Can you work these out from the model? Positions are in its coordinate system, mm. A direction names the side the tool comes from. Give positions to 0.01 mm unless a question says otherwise; leave off trailing zeros. Write each loop counter-clockwise with the first axis right and the second up, starting at its lowest first coordinate (ties: lowest second). Pieces come first, ordered by that corner, then holes.
```python
from build123d import *

# Parameters (mm, degrees)
SKETCH1_W               = 240
SKETCH1_H               = 20
BOSS_EXTRUDE1_DEPTH     = 30
SKETCH2_R               = 5.025
CUT_EXTRUDE1_DEPTH      = 20
SKETCH3_R               = 2.05
CUT_EXTRUDE2_DEPTH      = 30
SKETCH4_W               = 15
SKETCH4_H               = 30
CUT_EXTRUDE3_DEPTH      = 10
CUT_EXTRUDE4_DEPTH      = 2.5
CUT_EXTRUDE5_DEPTH      = 32.5
FILLET1_R               = 10
FILLET2_R               = 10
CHAMFER1_SIZE           = 1
CHAMFER2_SIZE           = 1
SKETCH7_R               = 1.6
CUT_EXTRUDE6_DEPTH      = 32.5
CUT_EXTRUDE7_DEPTH      = 10
SKETCH9_R               = 3
CUT_EXTRUDE8_DEPTH      = 3
FILLET3_R               = 1
CUT_EXTRUDE9_DEPTH      = 3
CUT_EXTRUDE9_DEPTH_BACK = 3
SKETCH10_R              = 3.65
SKETCH11_R              = 1.5
CUT_EXTRUDE10_DEPTH     = 13
SKETCH12_R              = 2.75
SKETCH12_R_2            = 1.5
CUT_EXTRUDE11_DEPTH     = 3


with BuildPart() as part:
    # Sketch1 → Boss-Extrude1 (new body)
    with BuildSketch(Plane(origin=(0, 0, 0), x_dir=(0, 0, -1), z_dir=(1, 0, 0))):
        with Locations((47.599764496, 4.521643901)):
            Rectangle(SKETCH1_W, SKETCH1_H)
    extrude(amount=BOSS_EXTRUDE1_DEPTH)

    # Sketch2 → Cut-Extrude1 (cut)
    with BuildSketch(Plane(origin=(0, 14.521643901, 0), x_dir=(1, 0, 0), z_dir=(0, 1, 0))):
        with Locations(Location((15, 147.599764496, 0), (0, 0, 270))):
            Circle(SKETCH2_R)
        with Locations(Location((15, -52.400235504, 0), (0, 0, 270))):
            Circle(SKETCH2_R)
    extrude(amount=-CUT_EXTRUDE1_DEPTH, mode=Mode.SUBTRACT)

    # Sketch3 → Cut-Extrude2 (cut)
    with BuildSketch(Plane(origin=(30, 0, 0), x_dir=(0, 0, -1), z_dir=(1, 0, 0))):
        with Locations((117.599764496, 4.521643901)):
            Circle(SKETCH3_R)
        with Locations((-22.400235504, 4.521643901)):
            Circle(SKETCH3_R)
        with Locations((12.599764496, 4.521643901)):
            Circle(SKETCH3_R)
        with Locations((82.599764496, 4.521643901)):
            Circle(SKETCH3_R)
    extrude(amount=-CUT_EXTRUDE2_DEPTH, mode=Mode.SUBTRACT)

    # Sketch4 → Cut-Extrude3 (cut)
    with BuildSketch(Plane(origin=(0, 14.521643901, 0), x_dir=(1, 0, 0), z_dir=(0, 1, 0))):
        with Locations((15, 47.599764496)):
            Rectangle(SKETCH4_W, SKETCH4_H)
    extrude(amount=-CUT_EXTRUDE3_DEPTH, mode=Mode.SUBTRACT)

    # Sketch5 → Cut-Extrude4 (cut)
    with BuildSketch(Plane(origin=(0, 4.521643901, 0), x_dir=(1, 0, 0), z_dir=(0, 1, 0))):
        Polygon((15, 44.424338015), (17.75, 46.012051256), (17.75, 49.187477736), (15, 50.775190977), (12.25, 49.187477736), (12.25, 46.012051256), align=None)
    extrude(amount=-CUT_EXTRUDE4_DEPTH, mode=Mode.SUBTRACT)

    # Sketch6 → Cut-Extrude5 (cut)
    with BuildSketch(Plane.XZ.offset(5.478356099)):
        Polygon((30, 37.400235504), (20, 25.482699578), (20, -14.517300422), (30, -26.434836348), align=None)
        Polygon((30, -68.764692644), (20, -80.68222857), (20, -120.68222857), (30, -132.599764496), align=None)
    extrude(amount=-CUT_EXTRUDE5_DEPTH, mode=Mode.SUBTRACT)

    # Fillet1
    fillet1_edges = [part.edges().sort_by_distance(p)[0] for p in [
        (30, 4.521643901, -68.764692644),
        (30, 4.521643901, -26.434836348),
    ]]
    fillet(fillet1_edges, radius=FILLET1_R)

    # Fillet2
    fillet2_edges = [part.edges().sort_by_distance(p)[0] for p in [
        (30, 4.521643901, -132.599764496),
        (30, 4.521643901, 72.400235504),
        (30, 4.521643901, -167.599764496),
        (30, 4.521643901, 37.400235504),
    ]]
    fillet(fillet2_edges, radius=FILLET2_R)

    # Chamfer1
    chamfer1_edges = [part.edges().sort_by_distance(p)[0] for p in [
        (20, -5.478356099, -100.68222857),
        (23.830222216, -5.478356099, -125.246909656),
        (30, -5.478356099, -47.599764496),
        (23.830222216, -5.478356099, -76.117547484),
        (29.396926208, -5.478356099, -68.545191735),
        (29.396926208, -5.478356099, -26.654337257),
        (30, -5.478356099, 51.720086675),
        (23.830222216, -5.478356099, 30.047380664),
        (10, -5.478356099, 72.400235504),
        (10, -5.478356099, -167.599764496),
        (30, -5.478356099, -146.919615667),
        (29.396926208, -5.478356099, 37.619736413),
        (29.396926208, -5.478356099, -132.819265405),
        (27.071067812, -5.478356099, -164.670832308),
        (27.071067812, -5.478356099, 69.471303316),
        (20, -5.478356099, 5.482699578),
        (23.830222216, -5.478356099, -19.081981508),
    ]]
    chamfer(chamfer1_edges, length=CHAMFER1_SIZE)

    # Chamfer2
    chamfer2_edges = [part.edges().sort_by_distance(p)[0] for p in [
        (23.830222216, 14.521643901, -125.246909656),
        (20, 14.521643901, -100.68222857),
        (30, 14.521643901, -47.599764496),
        (23.830222216, 14.521643901, -76.117547484),
        (29.396926208, 14.521643901, -68.545191735),
        (29.396926208, 14.521643901, -26.654337257),
        (30, 14.521643901, 51.720086675),
        (10, 14.521643901, 72.400235504),
        (30, 14.521643901, -146.919615667),
        (10, 14.521643901, -167.599764496),
        (23.830222216, 14.521643901, 30.047380664),
        (29.396926208, 14.521643901, 37.619736413),
        (29.396926208, 14.521643901, -132.819265405),
        (27.071067812, 14.521643901, -164.670832308),
        (27.071067812, 14.521643901, 69.471303316),
        (23.830222216, 14.521643901, -19.081981508),
        (20, 14.521643901, 5.482699578),
    ]]
    chamfer(chamfer2_edges, length=CHAMFER2_SIZE)

    # Sketch7 → Cut-Extrude6 (cut)
    with BuildSketch(Plane(origin=(0, 2.021643901, 0), x_dir=(1, 0, 0), z_dir=(0, 1, 0))):
        with Locations(Location((15, 47.599764496, 0), (0, 0, 270))):
            Circle(SKETCH7_R)
    extrude(amount=-CUT_EXTRUDE6_DEPTH, mode=Mode.SUBTRACT)

    # Sketch8 → Cut-Extrude7 (cut)
    with BuildSketch(Plane(origin=(0, 14.521643901, 0), x_dir=(1, 0, 0), z_dir=(0, 1, 0))):
        Polygon((7.5, 65.599764496), (8.75, 62.599764496), (21.25, 62.599764496), (22.5, 65.599764496), align=None)
        Polygon((21.25, 32.599764496), (8.75, 32.599764496), (7.5, 29.599764496), (22.5, 29.599764496), align=None)
    extrude(amount=-CUT_EXTRUDE7_DEPTH, mode=Mode.SUBTRACT)

    # Sketch9 → Cut-Extrude8 (cut)
    with BuildSketch(Plane.XZ.offset(5.478356099)):
        with Locations(Location((15, -47.599764496, 0), (0, 0, 270))):
            Circle(SKETCH9_R)
    extrude(amount=-CUT_EXTRUDE8_DEPTH, mode=Mode.SUBTRACT)

    # Fillet3
    fillet3_edges = [part.edges().sort_by_distance(p)[0] for p in [
        (15, -5.478356099, -44.599764496),
    ]]
    fillet(fillet3_edges, radius=FILLET3_R)

    # Sketch10 → Cut-Extrude9 (cut, two sides: drawn at the far end of the back side and taken through both)
    with BuildSketch(Plane(origin=(20, 0, 0), x_dir=(0, 0, -1), z_dir=(1, 0, 0)).offset(-CUT_EXTRUDE9_DEPTH_BACK)):
        with Locations(Location((12.599764496, 4.521643901, 0), (0, 0, 301.691963515))):
            Circle(SKETCH10_R)
        with Locations(Location((-22.400235504, 4.521643901, 0), (0, 0, 147.61954983))):
            Circle(SKETCH10_R)
        with Locations(Location((82.599764496, 4.521643901, 0), (0, 0, 238.308036485))):
            Circle(SKETCH10_R)
        with Locations(Location((117.599764496, 4.521643901, 0), (0, 0, 327.61954983))):
            Circle(SKETCH10_R)
    extrude(amount=CUT_EXTRUDE9_DEPTH + CUT_EXTRUDE9_DEPTH_BACK, mode=Mode.SUBTRACT)

    # Sketch11 → Cut-Extrude10 (cut)
    with BuildSketch(Plane(origin=(30, 0, 0), x_dir=(0, 0, -1), z_dir=(1, 0, 0))):
        with Locations((147.599764496, 4.521643901)):
            Circle(SKETCH11_R)
        with Locations((-52.400235504, 4.521643901)):
            Circle(SKETCH11_R)
    extrude(amount=-CUT_EXTRUDE10_DEPTH, mode=Mode.SUBTRACT)

    # Sketch12 → Cut-Extrude11 (cut)
    # profile 1 of 2: a face of its own
    with BuildSketch(Plane(origin=(30, 0, 0), x_dir=(0, 0, -1), z_dir=(1, 0, 0))):
        with Locations((-52.400235504, 4.521643901)):
            Circle(SKETCH12_R)
        with Locations((-52.400235504, 4.521643901)):
            Circle(SKETCH12_R_2, mode=Mode.SUBTRACT)
    # profile 2 of 2: a face of its own
    with BuildSketch(Plane(origin=(30, 0, 0), x_dir=(0, 0, -1), z_dir=(1, 0, 0))):
        with Locations((147.599764496, 4.521643901)):
            Circle(SKETCH12_R)
        with Locations((147.599764496, 4.521643901)):
            Circle(SKETCH12_R_2, mode=Mode.SUBTRACT)
    extrude(amount=-CUT_EXTRUDE11_DEPTH, mode=Mode.SUBTRACT)


solid = part.part
```
1) For pin 1 Ø1.8 at (y, z) = (4.52, -147.6) entering from +X; pin 2 Ø3.5 at (x, z) = (15, -47.6) entering from -Y; pin 3 Ø0.6 at (x, y) = (22, 10.5) entering from +Z, each with a flat end and sliding along its axis, tell me the tip position at first contact or that it passes through.
Values follow:
pin 1: stops at x = 10.06
pin 2: stops at y = -2.48
pin 3: stops at z = 72.25
2) Suppose I cut it at B-B on z = -92. Write out the boundary of the cut face in (x, y).
Values follow:
outline: (0, -5.48) - (19, -5.48) - (20, -4.48) - (20, 13.52) - (19, 14.52) - (0, 14.52) - close
3) If we mould it in two halves opening along Z, with no side actions, what happens to faces 1 (the face through (13.85, -3.49, -50.37)), 2 (the face through (30, 5, -144)), 3 (the face through (10, 4, 72.4))? For each: +Z half, -Z half, draft (parallel to the pull), parting line (faces both ways), or undercut.
Values follow:
face 1: undercut
face 2: draft
face 3: +Z half
4) Please list where these lines run through material, in increasing order: L1, parallel to Z at x = 15.25, y = 8; L2, parallel to Z at x = 2, y = 4.25; L3, parallel to X at y = 6, z = -147.
Values follow:
L1: z = -167.6 to -152.62, -142.58 to -65.6, -29.6 to 47.38, 57.42 to 72.4
L2: z = -167.6 to -119.63, -115.57 to -84.63, -80.57 to -14.63, -10.57 to 20.37, 24.43 to 72.4
L3: x = 0 to 10.01, 19.99 to 27
5) For faces 4 (the face through (18.79, 4.47, -16.25)), 5 (the face through (23, 14, -125)), 6 (the face through (23.884, 4.396, -76.054)), which set-ups out of +Z, -Z, +X, -X, +Y, -Y let a thin tool reach every point of the face, with its end or its side?
Values follow:
face 4: +X
face 5: +X, +Y
face 6: +X, +Y, -Y
6) Suppose I cut it at A-A on z = -117.5. Write out the boundary of the cut face in (x, y).
Values follow:
outline: (0, -5.48) - (19, -5.48) - (20, -4.48) - (20, 0.87) - (17, 0.87) - (17, 2.47) - (0, 2.47) - close; (0, 6.57) - (17, 6.57) - (17, 8.17) - (20, 8.17) - (20, 13.52) - (19, 14.52) - (0, 14.52) - close
